Source: three-view drawing plus pictorial views. Frame: mm from the lowest corner of the part. A direction names the side the tool comes from. Coordinates: 2 decimals unless noted, no trailing zeros. Loops run counter-clockwise (first coordinate to the right, second up) from the corner with the lowest first, then second, coordinate; pieces in that order, holes last.
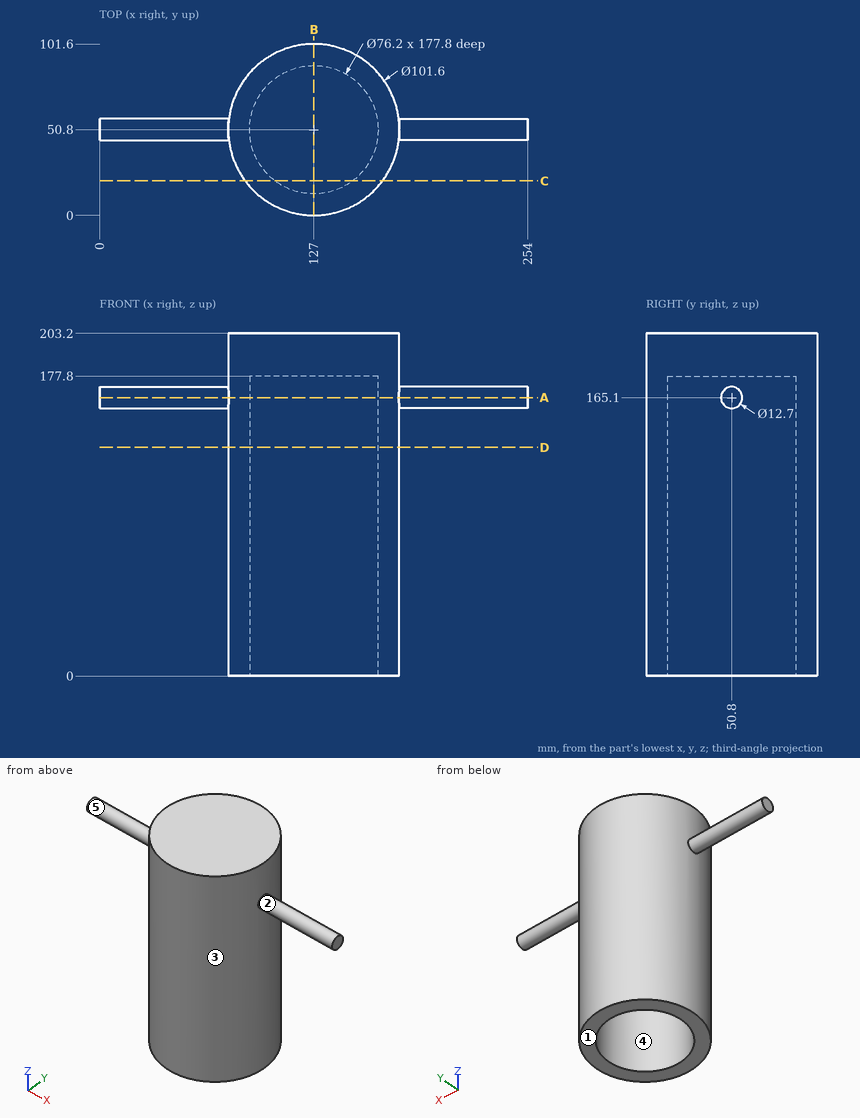
Q1. Access query for the marked faces 1 and 2. Directions: +Z, -Z, +X, -X, +Y, -Y. A direction counts if a zero-diameter tool reaches every point of the face in a straight line with its end or side. Return the directions, or none.
Q2. Section B-B, the plane x = 127. Return the cut outline in (y, z), plus the area to 3 significant figures.
Q3. Line query: line 1 along X through (y, z) = (50, 129); line 2 along Y through (x, z) = (126.5, 56.5); line 3 along Z through (x, y) = (160.5, 66). Output: solid intervals per line, ascending.
Q4. Section D-D, the plane z = 135.5. Return the cut outline in (x, y).
Q5. Draft query along X for the marked faces 3, 4 and 5. Return one class per face: +X half, -X half, draft (parallel to the pull), parting line (faces both ways), or undercut.
Q6. Contact query for flat-ended pins moving along their axis: pin 1 Ø1.5 at (x, z) = (169.5, 45) entering from +Y; pin 2 Ø10 at (y, z) = (33.5, 74) entering from -X; pin 3 Ø5 at (x, y) = (210.5, 50) entering from -Z. Output: stop coordinate, or through.
Q7. Section A-A, the plane z = 165.1. Return the cut outline in (x, y), plus the area to 3 significant figures.
Q8. Section C-C, the plane y = 20.5. Return the cut outline in (x, z), plus the area to 3 significant figures.
Derived:
1. face 1: -Z, +X, -X, +Y, -Y
1. face 2: +X
2. outline: (0, 0) - (12.7, 0) - (12.7, 177.8) - (88.9, 177.8) - (88.9, 0) - (101.6, 0) - (101.6, 203.2) - (0, 203.2) - close
2. area: 7,100 mm2
3. line 1: x = 76.21 to 88.91, 165.09 to 177.79
3. line 2: y = 0 to 12.7, 88.9 to 101.6
3. line 3: z = 177.8 to 203.2
4. outline: circle Ø101.6 at (127, 50.8); hole circle Ø76.2 at (127, 50.8)
5. face 3: parting line
5. face 4: undercut
5. face 5: draft
6. pin 1: stops at y = 79.74
6. pin 2: stops at x = 77.71
6. pin 3: stops at z = 158.75
7. outline: (0, 44.45) - (76.6, 44.45) arc R50.8 ccw to (177.4, 44.45) - (254, 44.45) - (254, 57.15) - (177.4, 57.15) arc R50.8 ccw to (76.6, 57.15) - (0, 57.15) - close; hole circle Ø76.2 at (127, 50.8)
7. area: 5,490 mm2
8. outline: (86.23, 0) - (103.9, 0) - (103.9, 177.8) - (150.1, 177.8) - (150.1, 0) - (167.77, 0) - (167.77, 203.2) - (86.23, 203.2) - close
8. area: 8,360 mm2
